Answer from the drawing. Dimensions are ordinates in mm from the lowest x, y and z of the part. A direction names the side the tool comes from. Round coordinates to 2 decimals unless told otherwise and drop trailing zeros. Loops run counter-clockwise (first coordinate to the right, second up) from the corner with the lowest first, then second, coordinate; pieces in that order, holes last. Notation, with made-up numbers: M -20,-24.5 L -9,-24.5 A7 ccw -9,-15.5 Z; hole C 85.25,-19.5 d4. An arc over 180 degrees is marked long. One line per item, written item: value.
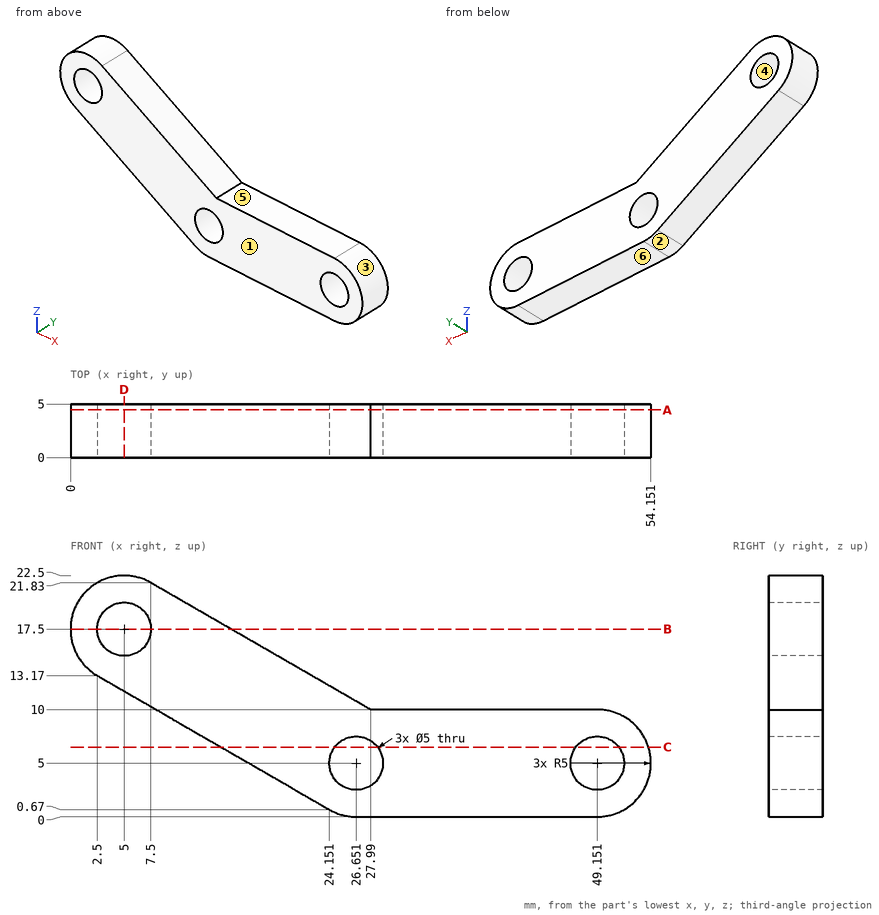
1) Find the intervals of material crossed by probe 1 along X at (y, z) = (1.6, 4.75) (1 decimal); probe 2 along X at (y, z) = (3.2, 5); probe 3 along X at (y, z) = (4, 17.5), in increasing order. Write a range as from..to.
Check values:
probe 1: 17.1..24.2, 29.1..46.7, 51.6..54.1
probe 2: 16.65..24.15, 29.15..46.65, 51.65..54.15
probe 3: 0..2.5, 7.5..15
2) Find section D-D (x = 5). Give the vertices of the cut face in (y, z).
Check values:
outline: M 0,11.73 L 5,11.73 L 5,15 L 0,15 Z; M 0,20 L 5,20 L 5,22.5 L 0,22.5 Z
3) Find section B-B (z = 17.5). Give the vertices of the cut face in (x, y).
Check values:
outline: M 0,0 L 2.5,0 L 2.5,5 L 0,5 Z; M 7.5,0 L 15,0 L 15,5 L 7.5,5 Z
4) For the marked faces 5 and 6, determine the directions among +Z, -Z, +X, -X, +Y, -Y from which every point of the face is accessible in a straight line to the end or side of a thin tool.
Check values:
face 5: +Z, +X, +Y, -Y
face 6: -Z, +X, -X, +Y, -Y
5) Find section C-C (z = 6.5). Give the vertices of the cut face in (x, y), then the cut area to 3 significant figures.
Check values:
outline: M 14.05,0 L 24.65,0 L 24.65,5 L 14.05,5 Z; M 28.65,0 L 47.15,0 L 47.15,5 L 28.65,5 Z; M 51.15,0 L 53.92,0 L 53.92,5 L 51.15,5 Z
area: 159 mm2
6) The mould has two halves that part along X. Classify the marked faces 1, 2, 3 and 4: +X half, -X half, draft (parallel to the pull), parting line (faces both ways), or undercut.
Check values:
face 1: draft
face 2: -X half
face 3: +X half
face 4: undercut
7) Find section A-A (y = 4.45). Give the vertices of the cut face in (x, z).
Check values:
outline: M 2.5,13.17 L 24.15,0.67 A5 ccw 26.65,0 L 49.15,0 A5 ccw 49.15,10 L 27.99,10 L 7.5,21.83 A5 ccw Z; hole C 5,17.5 d5; hole C 26.65,5 d5; hole C 49.15,5 d5
8) This flat-tipped pin is pushed along its axis until it touches: pin 1 (3 mm diameter, centred on x = 47.5, y = 2.5, fed in from +Z). Where does it stop, or does it pass through?
Check values:
pin 1: z = 10
